Design review of the part built by this model. Coordinates are the model's own, in mm. Give positions to 0.01 mm unless a question says otherwise; leave off trailing zeros. Loops run counter-clockwise (first coordinate to the right, second up) from the corner with the lowest first, then second, coordinate; pieces in that order, holes last. Notation, with made-up numbers: (-4, 3) -> (21, 3) arc R24 ccw to (21, 26) -> close; hole circle Ø9 at (20, 13.5). An arc over 180 degrees is marked (long way). Answer as CSV lines item,"result".
from build123d import *

# Parameters (mm, degrees)
SKETCH1_W           = 200
SKETCH1_H           = 84
SKETCH1_R           = 2.25
SKETCH1_R_2         = 2.5
BOSS_EXTRUDE1_DEPTH = 5
SKETCH2_W           = 200
SKETCH2_H           = 79
SKETCH2_R           = 2.25
BOSS_EXTRUDE2_DEPTH = 3
CHAMFER1_SIZE       = 8
CHAMFER3_SIZE       = 3
SKETCH3_W           = 7.071067812
SKETCH3_H           = 2.6
CUT_EXTRUDE1_DEPTH  = 234.034075139
SKETCH4_R           = 2.5
CUT_EXTRUDE2_DEPTH  = 218.071416819


with BuildPart() as part:
    # Sketch1 → Boss-Extrude1 (new body)
    with BuildSketch(Plane.XY):
        with Locations((100, 42)):
            Rectangle(SKETCH1_W, SKETCH1_H)
        with Locations((20, 9)):
            Circle(SKETCH1_R, mode=Mode.SUBTRACT)
        with Locations(Location((180, 9, 0), (0, 0, 180))):
            Circle(SKETCH1_R, mode=Mode.SUBTRACT)
        with Locations((20, 72)):
            Circle(SKETCH1_R, mode=Mode.SUBTRACT)
        with Locations(Location((180, 72, 0), (0, 0, 180))):
            Circle(SKETCH1_R, mode=Mode.SUBTRACT)
        with Locations((109.377508284, 51)):
            Circle(SKETCH1_R_2, mode=Mode.SUBTRACT)
        with Locations((129.377508284, 71)):
            Circle(SKETCH1_R_2, mode=Mode.SUBTRACT)
    extrude(amount=-BOSS_EXTRUDE1_DEPTH)

    # Sketch2 → Boss-Extrude2 (add)
    with BuildSketch(Plane(origin=(0, 0, -5), x_dir=(-1, 0, 0), z_dir=(0, 0, -1))):
        with Locations((-100, 44.5)):
            Rectangle(SKETCH2_W, SKETCH2_H)
        with Locations(Location((-20, 9, 0), (0, 0, 180))):
            Circle(SKETCH2_R, mode=Mode.SUBTRACT)
        with Locations((-180, 9)):
            Circle(SKETCH2_R, mode=Mode.SUBTRACT)
        with Locations(Location((-20, 72, 0), (0, 0, 180))):
            Circle(SKETCH2_R, mode=Mode.SUBTRACT)
        with Locations((-180, 72)):
            Circle(SKETCH2_R, mode=Mode.SUBTRACT)
    extrude(amount=BOSS_EXTRUDE2_DEPTH)

    # Chamfer1
    # the kernel refuses this chamfer: 8 mm, written as the material it takes off along each edge
    with BuildSketch(Plane(origin=(200, -15.573463904, -8), x_dir=(-0.9996219169112968, 0, -0.027495876610586296), z_dir=(0, 1, 0)), Plane(origin=(0, 104.573463904, -8), x_dir=(0.9996219169112968, 0, -0.027495876610586275), z_dir=(0, -1, 0))) as chamfer1_piece_1:
        Polygon((CHAMFER1_SIZE * 0.999621916911, CHAMFER1_SIZE * 0.0274958766106), (-CHAMFER1_SIZE * 0.0274958766106, CHAMFER1_SIZE * 0.999621916911), (0, 0), align=None)
    extrude(amount=120.146927807, mode=Mode.SUBTRACT)

    # Chamfer3
    chamfer3_edges = [part.edges().sort_by_distance(p)[0] for p in [
        (100, 84, -8),
    ]]
    chamfer(chamfer3_edges, length=CHAMFER3_SIZE)

    # Sketch3 → Cut-Extrude1 (cut, through all, along a direction that is not the sketch's normal)
    with BuildSketch(Plane(origin=(100, 0, -100), x_dir=(-0.7071067811865452, 0, -0.7071067811865498), z_dir=(0.7071067811865498, 0, -0.7071067811865452))):
        with Locations((-137.885822331, 1.3)):
            Rectangle(SKETCH3_W, SKETCH3_H)
    extrude(amount=-CUT_EXTRUDE1_DEPTH, dir=(1, 0, 0), mode=Mode.SUBTRACT)

    # Sketch4 → Cut-Extrude2 (cut, through all)
    with BuildSketch(Plane.XY):
        with Locations((129.377508284, 71)):
            Circle(SKETCH4_R)
        with Locations((109.377508284, 51)):
            Circle(SKETCH4_R)
    extrude(amount=-CUT_EXTRUDE2_DEPTH, mode=Mode.SUBTRACT)


solid = part.part
Q1. We need section A-A, the plane y = 9. State the section outline as (x, z) points.
Filled sheet:
outline,"(0, 0) -> (8, -8) -> (17.75, -8) -> (17.75, 0) -> close; (22.25, -8) -> (177.75, -8) -> (177.75, 0) -> (22.25, 0) -> close; (182.25, -8) -> (192, -8) -> (200, 0) -> (182.25, 0) -> close"
Q2. The part is to be moulded in two halves that separate along Y. For faces 1 (the flat face through (196, 43, -4)), 2 (the flat face through (97, 2.6, -4)), 3 (the flat face through (101, 84, -2)), say which applies: pulls with the +Y half, pulls with the -Y half, needs draft (parallel to the pull), parting line crosses it, or undercut.
Filled sheet:
face 1,"needs draft"
face 2,"pulls with the -Y half"
face 3,"pulls with the +Y half"
Q3. To check wall thickness, follow probe 1 along Y at (x, z) = (20, -2.55); probe 2 along Y at (x, z) = (180, -7.25); probe 3 along Y at (x, z) = (129, -1.75). State the ranges of each line that lie inside material, in increasing order. Write a range as from..to.
Filled sheet:
probe 1,"y = 2.6..6.75, 11.25..69.75, 74.25..84"
probe 2,"y = 5..6.75, 11.25..69.75, 74.25..81.75"
probe 3,"y = 2.6..68.53, 73.47..84"
Q4. We need section B-B, the plane x = 20. State the section outline as (y, z) points, and give its area (4 significant figures).
Filled sheet:
outline,"(2.6, -5) -> (5, -5) -> (5, -8) -> (6.75, -8) -> (6.75, 0) -> (2.6, 0) -> close; (11.25, -8) -> (69.75, -8) -> (69.75, 0) -> (11.25, 0) -> close; (74.25, -8) -> (81, -8) -> (84, -5) -> (84, 0) -> (74.25, 0) -> close"
area,"567.5 mm^2"
Q5. Clearance check with flat-ended pins moving along their axes: pin 1 Ø1.9 at (x, y) = (137.5, 4) entering from -Z; pin 2 Ø8 at (x, y) = (109.38, 51) entering from -Z; pin 3 Ø1.5 at (x, z) = (84, -6.5) entering from -Y; pin 4 Ø1 at (y, z) = (21.5, -3) entering from -X. State where each tip first meets the part, or that it passes through.
Filled sheet:
pin 1,"stops at z = -5"
pin 2,"stops at z = -8"
pin 3,"stops at y = 5"
pin 4,"stops at x = 2.5"
Q6. We need section D-D, the plane y = 51. State the section outline as (x, z) points.
Filled sheet:
outline,"(0, 0) -> (8, -8) -> (106.88, -8) -> (106.88, 0) -> close; (111.88, -8) -> (192, -8) -> (200, 0) -> (111.88, 0) -> close"
Q7. We need section C-C, the plane z = -3.25. State the section outline as (x, y) points, and give its area (3 significant figures).
Filled sheet:
outline,"(3.25, 2.6) -> (196.75, 2.6) -> (196.75, 84) -> (3.25, 84) -> close; hole circle Ø4.5 at (20, 9); hole circle Ø4.5 at (20, 72); hole circle Ø5 at (109.38, 51); hole circle Ø5 at (129.38, 71); hole circle Ø4.5 at (180, 9); hole circle Ø4.5 at (180, 72)"
area,"15,600 mm^2"
